```python
from build123d import *

# Parameters (mm, degrees)
SKETCH_1_R             = 12.5
EXTRUDE_1_DEPTH        = 7
SKETCH_2_R             = 14
EXTRUDE_2_DEPTH        = 10
SKETCH_3_R             = 23.5
EXTRUDE_3_DEPTH        = 4
HOLE_WIZARD_M3_1_D     = 2.5
HOLE_WIZARD_M3_1_DEPTH = 8.5
HOLE_WIZARD_M3_1_TIP   = 0.751075774
HOLE_WIZARD_M2_1_D     = 1.6
HOLE_WIZARD_M2_1_DEPTH = 6
HOLE_WIZARD_M2_1_TIP   = 0.480688495
SKETCH_14_R            = 15
EXTRUDE_4_DEPTH        = 4
SKETCH_15_R            = 13
EXTRUDE_5_DEPTH        = 4
SKETCH_16_R            = 12.5
EXTRUDE_6_DEPTH        = 4
SKETCH_4_R             = 9
CUT_EXTRUDE_2_DEPTH    = 47.834816109


with BuildPart() as part:
    # 草图1 → 凸台-拉伸1 (new body)
    with BuildSketch(Plane(origin=(0, 0, 0), x_dir=(0, 0, -1), z_dir=(1, 0, 0))):
        Circle(SKETCH_1_R)
    extrude(amount=EXTRUDE_1_DEPTH)

    # 草图2 → 凸台-拉伸2 (add)
    with BuildSketch(Plane(origin=(7, 0, 0), x_dir=(0, 0, -1), z_dir=(1, 0, 0))):
        Circle(SKETCH_2_R)
    extrude(amount=EXTRUDE_2_DEPTH)

    # 草图3 → 凸台-拉伸3 (add)
    with BuildSketch(Plane(origin=(17, 0, 0), x_dir=(0, 0, -1), z_dir=(1, 0, 0))):
        Circle(SKETCH_3_R)
    extrude(amount=EXTRUDE_3_DEPTH)

    # M3 螺纹孔1
    with Locations(Plane(origin=(21, 0, 0), x_dir=(0, 0, -1), z_dir=(1, 0, 0))):
        with Locations((0, 21), (21, 0), (0, -21), (-21, 0)):
            Hole(HOLE_WIZARD_M3_1_D / 2, depth=HOLE_WIZARD_M3_1_DEPTH)
            with Locations((0, 0, -(HOLE_WIZARD_M3_1_DEPTH + HOLE_WIZARD_M3_1_TIP / 2))):  # 118° drill point
                Cone(0, HOLE_WIZARD_M3_1_D / 2, HOLE_WIZARD_M3_1_TIP, mode=Mode.SUBTRACT)

    # M2 螺纹孔1
    with Locations(Plane.ZY):
        with Locations((-11, 0), (0, -11), (11, 0), (0, 11)):
            Hole(HOLE_WIZARD_M2_1_D / 2, depth=HOLE_WIZARD_M2_1_DEPTH)
            with Locations((0, 0, -(HOLE_WIZARD_M2_1_DEPTH + HOLE_WIZARD_M2_1_TIP / 2))):  # 118° drill point
                Cone(0, HOLE_WIZARD_M2_1_D / 2, HOLE_WIZARD_M2_1_TIP, mode=Mode.SUBTRACT)

    # 草图14 → 凸台-拉伸4 (add)
    with BuildSketch(Plane(origin=(21, 0, 0), x_dir=(0, 0, -1), z_dir=(1, 0, 0))):
        Circle(SKETCH_14_R)
    extrude(amount=EXTRUDE_4_DEPTH)

    # 草图15 → 凸台-拉伸5 (add)
    with BuildSketch(Plane(origin=(25, 0, 0), x_dir=(0, 0, -1), z_dir=(1, 0, 0))):
        Circle(SKETCH_15_R)
    extrude(amount=EXTRUDE_5_DEPTH)

    # 草图16 → 凸台-拉伸6 (add)
    with BuildSketch(Plane(origin=(29, 0, 0), x_dir=(0, 0, -1), z_dir=(1, 0, 0))):
        Circle(SKETCH_16_R)
    extrude(amount=EXTRUDE_6_DEPTH)

    # 草图4 → 切除-拉伸2 (cut, through all)
    with BuildSketch(Plane(origin=(0, 0, 0), x_dir=(0, 0, -1), z_dir=(1, 0, 0))):
        Circle(SKETCH_4_R)
    extrude(amount=CUT_EXTRUDE_2_DEPTH, mode=Mode.SUBTRACT)


solid = part.part
```
Can you work these out from the model? Positions are in its coordinate system, mm. A direction names the side the tool comes from. Give positions to 0.01 mm unless a question says otherwise; leave off trailing zeros. Loops run counter-clockwise (first coordinate to the right, second up) from the corner with the lowest first, then second, coordinate; pieces in that order, holes last. Notation, with made-up numbers: M 29,19.5 L 67,19.5 A14 cw 67,32.5 Z; hole C -3.5,43.25 d10. An arc over 180 degrees is marked long. Answer in a Markdown table with one row per item.
1. Suppose I cut it at C-C on x = 24. Write out the boundary of the cut face in (y, z).
Taken from the geometry:
| item | result |
|---|---|
| outline | C 0,0 d30; hole C 0,0 d18 |
2. If I drill on line 1 along Y through (x, z) = (3.5, 0); line 2 along X through (y, z) = (20, 12); line 3 along Z through (x, y) = (22.5, 7), over which ranges is the centre line in solid material (lowest first)?
Taken from the geometry:
| item | result |
|---|---|
| line 1 | y = -12.5 to -11.8, -10.2 to -9, 9 to 10.2, 11.8 to 12.5 |
| line 2 | x = 17 to 21 |
| line 3 | z = -13.27 to -5.66, 5.66 to 13.27 |
3. Thinking about a two-plate mould opening in Z: for faces 1 (the conical face through (6.397, -10.862, -0.018)), 2 (the cylindrical face through (19, 7.1, -22.4)), 3 (the flat face through (29, 10.7, 6.8)), which applies, released by +Z, released by -Z, zero draft, split by the parting line, or undercut?
Taken from the geometry:
| item | result |
|---|---|
| face 1 | undercut |
| face 2 | split by the parting line |
| face 3 | zero draft |
4. Suppose I cut it at B-B on z = 21. Write out the boundary of the cut face in (x, y), plus the area to 3 significant figures.
Taken from the geometry:
| item | result |
|---|---|
| outline | M 17,-10.55 L 21,-10.55 L 21,-1.25 L 17,-1.25 Z; M 17,1.25 L 21,1.25 L 21,10.55 L 17,10.55 Z |
| area | 74.4 mm² |
5. For pin 1 Ø4 at (y, z) = (0, -21) entering from -X; pin 2 Ø22.5 at (y, z) = (-7, 1) entering from -X; pin 3 Ø3 at (x, y) = (9, 9) entering from -Z; pin 4 Ø3 at (x, y) = (20, 15) entering from -Z, each with a flat end and sliding along its axis, tell me the tip position at first contact or that it passes through.
Taken from the geometry:
| item | result |
|---|---|
| pin 1 | stops at x = 17 |
| pin 2 | stops at x = 0 |
| pin 3 | stops at z = -11.82 |
| pin 4 | stops at z = -19.24 |
6. Suppose I cut it at A-A on y = 7.5. Write out the boundary of the cut face in (x, z), plus the area to 3 significant figures.
Taken from the geometry:
| item | result |
|---|---|
| outline | M 0,-10 L 7,-10 L 7,-11.82 L 17,-11.82 L 17,-22.27 L 21,-22.27 L 21,-12.99 L 25,-12.99 L 25,-10.62 L 29,-10.62 L 29,-10 L 33,-10 L 33,-4.97 L 0,-4.97 Z; M 0,4.97 L 33,4.97 L 33,10 L 29,10 L 29,10.62 L 25,10.62 L 25,12.99 L 21,12.99 L 21,22.27 L 17,22.27 L 17,11.82 L 7,11.82 L 7,10 L 0,10 Z |
| area | 495 mm² |
7. Which directions (+Z, -Z, +X, -X, +Y, -Y) give clear straight access to the entire face, cutting with the end or side of a thin tool? Please do faces 4 (the flat face through (25, 13.4, 0.1)), 5 (the cylindrical face through (3.042, 0.24, 10.237)), 6 (the cylindrical face through (18.97, 19.78, -0.27)).
Taken from the geometry:
| item | result |
|---|---|
| face 4 | +X |
| face 5 | -X |
| face 6 | +X, -X |
